```python
from build123d import *

# Parameters (mm, degrees)
BOSS_EXTRUDE1_DEPTH = 10
CUT_EXTRUDE1_DEPTH  = 1
CIRPATTERN1_COUNT   = 2
CIRPATTERN1_ANGLE   = 180
BOSS_EXTRUDE2_DEPTH = 1
CIRPATTERN2_COUNT   = 2
CIRPATTERN2_ANGLE   = 180
FILLET1_R           = 1.5
FILLET2_R           = 1
FILLET3_R           = 2
SKETCH5_R           = 1.7
CUT_EXTRUDE2_DEPTH  = 23.276669473
SKETCH6_R           = 1.75
BOSS_EXTRUDE3_DEPTH = 1


# Some blends are built 0.0001 mm under size
with BuildPart() as part:
    # Sketch1 → Boss-Extrude1 (new, symmetric)
    with BuildSketch(Plane.XY):
        Polygon((-12.5, -4), (-12.5, 0), (12.5, 0), (12.5, -4), (11.5, -4), (11.5, -1), (-11.5, -1), (-11.5, -4), align=None)
    extrude(amount=BOSS_EXTRUDE1_DEPTH, both=True)

    # Sketch3 → Cut-Extrude1 (cut)
    with BuildSketch(Plane(origin=(12.5, 0, 0), x_dir=(0, 0, -1), z_dir=(1, 0, 0))):
        with BuildLine():
            Line((-2, -3), (-2, -4))
            Line((-2, -4), (0, -4))
            Line((0, -4), (0, -3))
            ThreePointArc((0, -3), (-1, -2), (-2, -3))
        make_face()
    cut_extrude1 = extrude(amount=-CUT_EXTRUDE1_DEPTH, mode=Mode.SUBTRACT)

    # CirPattern1: Cut-Extrude1 ×2 about axis
    cirpattern1_axis = Axis((0, -50, 0), (0, 1, 0))
    for i in range(1, CIRPATTERN1_COUNT):
        add(cut_extrude1.rotate(cirpattern1_axis, i * CIRPATTERN1_ANGLE / (CIRPATTERN1_COUNT - 1)), mode=Mode.SUBTRACT)

    # Sketch4 → Boss-Extrude2 (add)
    with BuildSketch(Plane.XZ.offset(4)):
        Polygon((12.5, -10), (19.5, -10), (19.5, -3.5), (12.5, 0), align=None)
    boss_extrude2 = extrude(amount=-BOSS_EXTRUDE2_DEPTH)

    # CirPattern2: Boss-Extrude2 ×2 about axis
    cirpattern2_axis = Axis((0, 0, 0), (0, 1, 0))
    for i in range(1, CIRPATTERN2_COUNT):
        add(boss_extrude2.rotate(cirpattern2_axis, i * CIRPATTERN2_ANGLE / (CIRPATTERN2_COUNT - 1)))

    # Fillet1
    fillet1_edges = [part.edges().sort_by_distance(p)[0] for p in [
        (19.5, -3.5, -3.5),
        (19.5, -3.5, -10),
        (-19.5, -3.5, 3.5),
        (-19.5, -3.5, 10),
    ]]
    fillet(fillet1_edges, radius=FILLET1_R)

    # Fillet2
    # the kernel refuses this fillet: 1 mm, written as the material it adds along each edge
    with BuildSketch(Plane(origin=(11.5, -1, 10), x_dir=(0, -1, 0), z_dir=(0, 0, -1))) as fillet2_piece_1:
        with BuildLine():
            CenterArc((FILLET2_R, FILLET2_R), FILLET2_R, 180, 90)
            Line((0, FILLET2_R), (0, 0))
            Line((0, 0), (FILLET2_R, 0))
        make_face()
    extrude(amount=20)
    with BuildSketch(Plane(origin=(-11.5, -1, -10), x_dir=(1, 0, 0), z_dir=(0, 0, 1))) as fillet2_piece_2:
        with BuildLine():
            CenterArc((FILLET2_R, -FILLET2_R), FILLET2_R, 90, 90)
            Line((0, -FILLET2_R), (0, 0))
            Line((0, 0), (FILLET2_R, 0))
        make_face()
    extrude(amount=20)
    with BuildSketch(Plane(origin=(-12.5, -3, -2.5), x_dir=(0, 1, 0), z_dir=(0, 0, 1))) as fillet2_piece_3_section:
        with BuildLine():
            CenterArc((FILLET2_R, FILLET2_R), FILLET2_R, 180, 90)
            Line((0, FILLET2_R), (0, 0))
            Line((0, 0), (FILLET2_R, 0))
        make_face()
    fillet2_piece_3 = extrude(amount=12.5, mode=Mode.PRIVATE)
    fillet2_piece_3 = split(fillet2_piece_3, bisect_by=Plane(origin=(-14.699431135, -2.775586215, 1.099715568), z_dir=(0.44721359549996453, 0, 0.8944271909999126)), keep=Keep.TOP, mode=Mode.PRIVATE)
    add(fillet2_piece_3)
    with BuildSketch(Plane(origin=(12.5, -3, 2.5), x_dir=(1, 0, 0), z_dir=(0, 0, -1))) as fillet2_piece_4_section:
        with BuildLine():
            CenterArc((FILLET2_R, -FILLET2_R), FILLET2_R, 90, 90)
            Line((0, -FILLET2_R), (0, 0))
            Line((0, 0), (FILLET2_R, 0))
        make_face()
    fillet2_piece_4 = extrude(amount=12.5, mode=Mode.PRIVATE)
    fillet2_piece_4 = split(fillet2_piece_4, bisect_by=Plane(origin=(14.699431135, -2.775586215, -1.099715568), z_dir=(-0.44721359549995826, 0, -0.8944271909999157)), keep=Keep.TOP, mode=Mode.PRIVATE)
    add(fillet2_piece_4)

    # Fillet3
    fillet3_edges = [part.edges().sort_by_distance(p)[0] for p in [
        (-12.5, 0, 0),
        (12.5, 0, 0),
        (11.5, -4, -5),
        (-11.5, -4, 5),
    ]]
    fillet(fillet3_edges, radius=FILLET3_R - 0.0001)  # a hair under: the kernel refuses the full size

    # Sketch5 → Cut-Extrude2 (cut, through all)
    with BuildSketch(Plane(origin=(0, 0, 0), x_dir=(1, 0, 0), z_dir=(0, 1, 0))):
        with Locations(Location((16.5, 7, 0), (0, 0, 270))):
            Circle(SKETCH5_R)
        with Locations(Location((-16.5, -7, 0), (0, 0, 270))):
            Circle(SKETCH5_R)
    extrude(amount=-CUT_EXTRUDE2_DEPTH, mode=Mode.SUBTRACT)

    # Sketch6 → Boss-Extrude3 (add)
    with BuildSketch(Plane.XZ.offset(1)):
        with Locations(Location((7.7, 7.7, 0), (0, 0, 90))):
            Circle(SKETCH6_R)
        with Locations(Location((-7.7, -7.7, 0), (0, 0, 90))):
            Circle(SKETCH6_R)
    extrude(amount=BOSS_EXTRUDE3_DEPTH)


solid = part.part
```
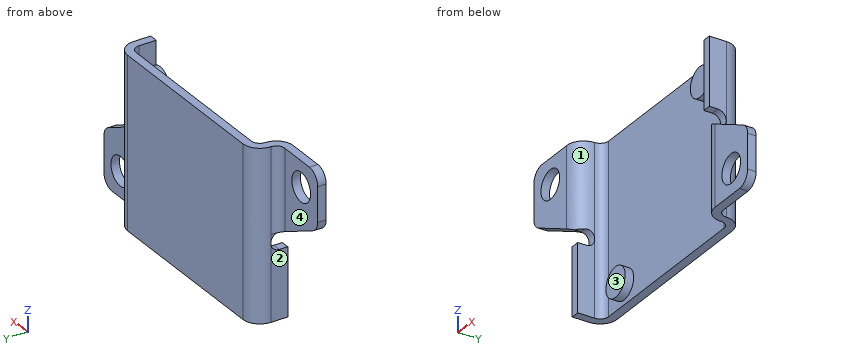
Can you work these out from the model? Positions are in its coordinate system, mm. Face numbers are marked on the shaded views. A direction names the side the tool comes from. Give positions to 0.01 mm unless a question says otherwise; leave off trailing zeros. Loops run counter-clockwise (first coordinate to the right, second up) from the corner with the lowest first, then second, coordinate; pieces in that order, holes last. Notation, with made-up numbers: M -18,-12.5 L 22,-12.5 A17 cw 22,16.5 Z; hole C 51,8.5 d4. An arc over 180 degrees is marked long. One line per item, written item: value.
(1) Suppose I cut it at D-D on x = -7. List the corners of the cut face in (y, z) for me, plus the area to 3 significant figures.
Returned:
outline: M -2,-9.3 L -1,-9.3 L -1,-10 L 0,-10 L 0,10 L -1,10 L -1,-6.1 L -2,-6.1 Z
area: 23.2 mm^2
(2) Will these pins go through, and if not, where does the flat tip stop? pin 1 (3 mm diameter, centred on x = 8, z = 7.5, fed in from -Y); pin 2 (1.5 mm diameter, centred on y = -1, z = 3, fed in from -X); pin 3 (4.5 mm diameter, centred on x = -16.5, z = 7, fed in from -Y); pin 4 (5 mm diameter, centred on x = 16.5, z = -4.5, fed in from +Y).
Returned:
pin 1: y = -2
pin 2: x = -12.48
pin 3: y = -4
pin 4: y = -3
(3) Suppose I cut it at A-A on x = 16.5. List the corners of the cut face in (y, z) for me.
Returned:
outline: M -4,-10 L -3,-10 L -3,-8.7 L -4,-8.7 Z; M -4,-5.3 L -3,-5.3 L -3,-2 L -4,-2 Z
(4) Which directions (+Z, -Z, +X, -X, +Y, -Y) give clear straight access to the entire face, cutting with the end or side of a thin tool? Please do the marked faces 1, 2, 3 and 4.
Returned:
face 1: +Z, -Y
face 2: -Z, -X, +Y, -Y
face 3: +Z, -Z, -Y
face 4: +Z, -Z, -X, +Y
(5) I need wall thicknesses on line 1 (X direction, y = -3.55, z = -7); line 2 (X direction, y = -3.8, z = -7); line 3 (X direction, y = -1.95, z = -4). Which ranges of each line are inside material? Lowest first, please.
Returned:
line 1: -12.5 to -11.5, 12.24 to 14.8, 18.2 to 19.5
line 2: -12.5 to -11.5, 12.63 to 14.8, 18.2 to 19.5
line 3: -12.5 to -11.5, 11.5 to 12.5
